Check sheet for the modelled part. Datum: model origin and axes. Units: mm. Face numbers are marked on the shaded views. A direction names the side the tool comes from. Give positions to 0.01 mm unless a question says otherwise; leave off trailing zeros. Order: outer loops, then holes, each group sorted by start corner. A loop starts at its lowest first (then second) coordinate and runs counter-clockwise, first axis right, second up.
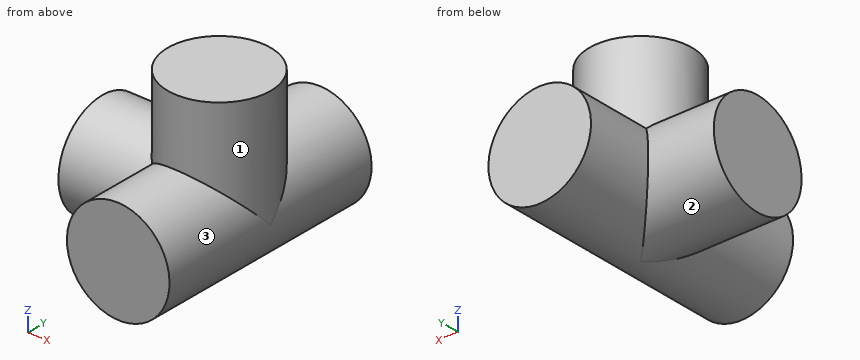
from build123d import *

# Parameters (mm, degrees)
CYLINDER015_R             = 13.9827
CYLINDER015_DEPTH         = 31.877
CYLINDER014_R             = 13.9827
CYLINDER014_DEPTH         = 64.36
CYLINDER016_R             = 13.9827
CYLINDER016_DEPTH         = 31.877
FUSION007_PLACEMENT_ANGLE = 90


with BuildPart() as cylinder015:
    # Cylinder015 → Cylinder015 (new body)
    with BuildSketch(Plane(origin=(0, 0, 0), x_dir=(0, 0, -1), z_dir=(1, 0, 0))):
        Circle(CYLINDER015_R)
    extrude(amount=CYLINDER015_DEPTH)


with BuildPart() as cylinder014:
    # Cylinder014 → Cylinder014 (new body)
    with BuildSketch(Plane.XZ.offset(-32.1818)):
        Circle(CYLINDER014_R)
    extrude(amount=CYLINDER014_DEPTH)


with BuildPart() as f_4_way001:
    # Cylinder016 → Cylinder016 (new body)
    with BuildSketch(Plane.XY):
        Circle(CYLINDER016_R)
    extrude(amount=CYLINDER016_DEPTH)

    # Fusion006: union Cylinder014
    add(cylinder014.part)

    # Fusion007: union Cylinder015
    add(cylinder015.part)


with BuildPart() as f_4_way001_1:
    # Fusion007 placement: moved
    add(f_4_way001.part.moved(Location((754, -15, 0))).rotate(Axis((754, -15, 0), (0, -1, 0)), FUSION007_PLACEMENT_ANGLE))


solid = f_4_way001_1.part
1) Section check B-B, the plane z = -8.5. Record the cut outline in (x, y).
Recorded:
outline: (722.12, -26.1) - (742.9, -26.1) - (742.9, -47.18) - (765.1, -47.18) - (765.1, 17.18) - (742.9, 17.18) - (742.9, -3.9) - (722.12, -3.9) - close
2) Section check C-C, the plane x = 750. Record the cut outline in (y, z).
Recorded:
outline: (-47.18, -13.4) - (-19, -13.4) arc R13.98 ccw to (-11, -13.4) - (17.18, -13.4) - (17.18, 13.4) - (-1.6, 13.4) - (-1.6, 31.88) - (-28.4, 31.88) - (-28.4, 13.4) - (-47.18, 13.4) - close
3) Section check A-A, the plane y = -15. Record the cut outline in (x, z).
Recorded:
outline: (722.12, -13.98) - (754, -13.98) arc R13.98 ccw to (767.98, 0) - (767.98, 31.88) - (740.02, 31.88) - (740.02, 13.98) - (722.12, 13.98) - close
4) Set-up check for the marked faces 1, 2 and 3: record each of +Z, -Z, +X, -X, +Y, -Y from which the full face is reachable in a straight line by a thin tool's end or side.
Recorded:
face 1: +Z
face 2: -X
face 3: none
5) Depth check by flat-ended pin: pin 1 Ø1.5 at (x, y) = (757.5, 8.5) entering from -Z; pin 2 Ø5 at (x, z) = (745.5, 26.5) entering from +Y; pin 3 Ø1 at (x, y) = (756.5, 10) entering from +Z. Enter the tip coordinate at first touch or a pass-through.
Recorded:
pin 1: stops at z = -13.71
pin 2: stops at y = -2.37
pin 3: stops at z = 13.84
6) Section check D-D, the plane z = 25.5. Record the cut outline in (x, y), then the cut area to 3 significant figures.
Recorded:
outline: circle Ø27.97 at (754, -15)
area: 614 mm2
7) Material ranges on L1, parallel to Y at x = 737.5, z = 0; L2, parallel to X at y = -14.5, z = 12; L3, parallel to X at y = 11.5, z = 7, recorded low to high.
Recorded:
L1: y = -28.98 to -1.02
L2: x = 722.12 to 767.97
L3: x = 741.9 to 766.1
